```python
from build123d import *

# Parameters (mm, degrees)
BOSS_EXTRUDE1_DEPTH = 20
SHELL1_T            = -2
RIB1_START          = -18
RIB1_DEPTH          = 18


# Read off the part's stored shape, not the designer's step: Rib1
with BuildPart() as part:
    # Sketch1 → Boss-Extrude1 (new body)
    with BuildSketch(Plane(origin=(0, 0, 0), x_dir=(1, 0, 0), z_dir=(0, 1, 0))):
        with BuildLine():
            Line((50, 30), (-55, 30))
            ThreePointArc((-55, 30), (-58.535533906, 28.535533906), (-60, 25))
            Line((-60, 25), (-60, -20))
            ThreePointArc((-60, -20), (-57.071067812, -27.071067812), (-50, -30))
            Line((-50, -30), (55, -30))
            ThreePointArc((55, -30), (58.535533906, -28.535533906), (60, -25))
            Line((60, -25), (60, 20))
            ThreePointArc((60, 20), (57.071067812, 27.071067812), (50, 30))
        make_face()
    extrude(amount=BOSS_EXTRUDE1_DEPTH)

    # Shell1
    shell1_openings = [part.faces().sort_by_distance(p)[0] for p in [
        (0, 20, 0),
    ]]
    offset(amount=SHELL1_T, openings=shell1_openings, kind=Kind.INTERSECTION)

    # Rib1 outline → Rib1 (add)
    with BuildSketch(Plane(origin=(0, 20, 0), x_dir=(1, 0, 0), z_dir=(0, 1, 0)).offset(RIB1_START)):
        with BuildLine():
            ThreePointArc((-1, 8.440971508), (-6.01040764, 6.01040764), (-8.440971508, 1))
            Line((-8.440971508, 1), (-58, 1))
            Line((-58, 1), (-58, -1))
            Line((-58, -1), (-8.440971508, -1))
            ThreePointArc((-8.440971508, -1), (-6.01040764, -6.01040764), (-1, -8.440971508))
            Line((-1, -8.440971508), (-1, -28))
            Line((-1, -28), (1, -28))
            Line((1, -28), (1, -8.440971508))
            ThreePointArc((1, -8.440971508), (6.01040764, -6.01040764), (8.440971508, -1))
            Line((8.440971508, -1), (58, -1))
            Line((58, -1), (58, 1))
            Line((58, 1), (8.440971508, 1))
            ThreePointArc((8.440971508, 1), (6.01040764, 6.01040764), (1, 8.440971508))
            Line((1, 8.440971508), (1, 28))
            Line((1, 28), (-1, 28))
            Line((-1, 28), (-1, 8.440971508))
        make_face()
        with BuildLine():
            Line((-1, -1), (-1, -6.422616289))
            ThreePointArc((-1, -6.422616289), (-4.596194078, -4.596194078), (-6.422616289, -1))
            Line((-6.422616289, -1), (-1, -1))
        make_face(mode=Mode.SUBTRACT)
        with BuildLine():
            Line((1, -1), (6.422616289, -1))
            ThreePointArc((6.422616289, -1), (4.596194078, -4.596194078), (1, -6.422616289))
            Line((1, -6.422616289), (1, -1))
        make_face(mode=Mode.SUBTRACT)
        with BuildLine():
            Line((-1, 1), (-6.422616289, 1))
            ThreePointArc((-6.422616289, 1), (-4.596194078, 4.596194078), (-1, 6.422616289))
            Line((-1, 6.422616289), (-1, 1))
        make_face(mode=Mode.SUBTRACT)
        with BuildLine():
            Line((1, 1), (1, 6.422616289))
            ThreePointArc((1, 6.422616289), (4.596194078, 4.596194078), (6.422616289, 1))
            Line((6.422616289, 1), (1, 1))
        make_face(mode=Mode.SUBTRACT)
    extrude(amount=RIB1_DEPTH)


solid = part.part
```
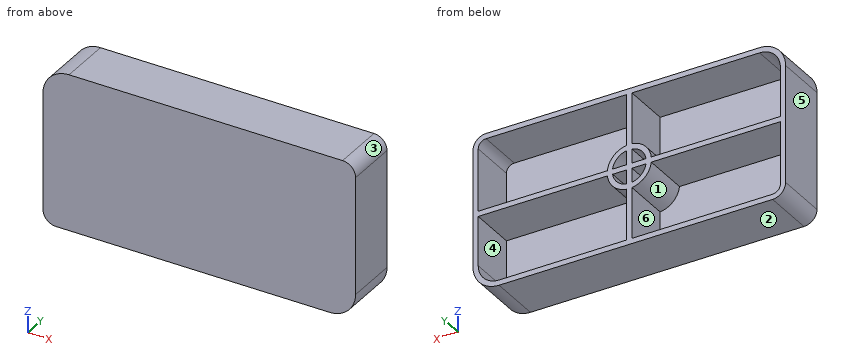
Check sheet for the modelled part. Datum: model origin and axes. Units: mm. Face numbers are marked on the shaded views. A direction names the side the tool comes from. Round coordinates to 2 decimals unless told otherwise and drop trailing zeros. Write each loop counter-clockwise with the first axis right and the second up, starting at its lowest first coordinate (ties: lowest second). Pieces come first, ordered by that corner, then holes. Notation, with made-up numbers: (52, 77) -> (110, 77) arc R18 cw to (110, 90) -> close; hole circle Ø4 at (11.5, 61.5). An arc over 180 degrees is marked (long way). Put each result on its own line as item: value.
(1) Material ranges on line 1 (X direction, y = 15.5, z = -19.5); line 2 (Z direction, x = -19.5, y = 18); line 3 (X direction, y = 7.25, z = -3), recorded low to high.
Values found:
line 1: x = -60 to -58, -1 to 1, 58 to 60
line 2: z = -30 to -28, -1 to 1, 28 to 30
line 3: x = -60 to -58, -7.95 to -5.77, -1 to 1, 5.77 to 7.95, 58 to 60
(2) Tool access check on the marked faces 5 and 6. Record the directions out of +Z, -Z, +X, -X, +Y, -Y that give a thin tool (end or side, any length) a straight path to the whole face; none if there is none.
Values found:
face 5: +Z, -Z, -X, +Y, -Y
face 6: +Y
(3) Go/stop test with flat-tipped pins: pin 1 Ø4.5 at (x, z) = (-2.5, 3) entering from +Y; pin 2 Ø13.5 at (x, z) = (-33, -15.5) entering from +Y. Record where each tip stops, or that it passes through.
Values found:
pin 1: stops at y = 20
pin 2: stops at y = 2
(4) Sectioned sample at D-D (z = 4.5). Enter the section's corners in (x, y).
Values found:
outline: (-60, 0) -> (60, 0) -> (60, 20) -> (58, 20) -> (58, 2) -> (7.21, 2) -> (7.21, 20) -> (4.69, 20) -> (4.69, 2) -> (1, 2) -> (1, 20) -> (-1, 20) -> (-1, 2) -> (-4.69, 2) -> (-4.69, 20) -> (-7.21, 20) -> (-7.21, 2) -> (-58, 2) -> (-58, 20) -> (-60, 20) -> close
(5) Sectioned sample at C-C (y = 17.75). Count the separate pieces of the cut face and the enclosed holes in it, plus the area to 3 significant figures.
Values found:
separate pieces: 1
enclosed holes: 8
area: 1,100 mm^2
(6) Sectioned sample at A-A (x = 12). Enter the section's corners in (y, z), plus the area to 3 significant figures.
Values found:
outline: (0, -30) -> (20, -30) -> (20, -28) -> (2, -28) -> (2, -1) -> (20, -1) -> (20, 1) -> (2, 1) -> (2, 28) -> (20, 28) -> (20, 30) -> (0, 30) -> close
area: 228 mm^2
(7) Mould release check, pull along X, two halves, no side actions. Record for the marked faces 1, 2, 3 and 4: released by +X, released by -X, zero draft, split by the parting line, or undercut.
Values found:
face 1: undercut
face 2: zero draft
face 3: released by +X
face 4: undercut
(8) Sectioned sample at B-B (z = -14). Enter the section's corners in (x, y), plus the area to 3 significant figures.
Values found:
outline: (-60, 0) -> (60, 0) -> (60, 20) -> (58, 20) -> (58, 2) -> (1, 2) -> (1, 20) -> (-1, 20) -> (-1, 2) -> (-58, 2) -> (-58, 20) -> (-60, 20) -> close
area: 348 mm^2
